from build123d import *

# Parameters (mm, degrees)
F0_R     = 3.675
F0_R_2   = 3.175
F1_DEPTH = 2.38125
F0_R_3   = 6.35
F0_R_4   = 5.85
F3_R     = 5.85
F3_R_2   = 3.675
F4_DEPTH = 0.25


# Not quite as in the source:
# - a length typed as a fraction of an inch, garbled in the dataset ("3 / 203.2 mm" for 3/8 in), is restored


with BuildPart() as f1:
    # F0 (on Top) → F1 (new body, symmetric)
    with BuildSketch(Plane.XY):
        Circle(F0_R)
        Circle(F0_R_2, mode=Mode.SUBTRACT)
    extrude(amount=F1_DEPTH, both=True)



with BuildPart() as f1b:
    # F0 (on Top) → F1, piece 2 (new body, symmetric)
    with BuildSketch(Plane.XY):
        Circle(F0_R_3)
        Circle(F0_R_4, mode=Mode.SUBTRACT)
    extrude(amount=F1_DEPTH, both=True)


with BuildPart() as f1_1:
    add(f1.part)

    add(f1b.part)  # F4 merges F1b
    # F3 (on offset) → F4 (join)
    with BuildSketch(Plane.XY.offset(1.88125)):
        Circle(F3_R)
        Circle(F3_R_2, mode=Mode.SUBTRACT)
    extrude(amount=F4_DEPTH)

    # F5: F1 across plane


with BuildPart() as f1_2:
    add(f1_1.part)
    add(f1_1.part.mirror(Plane.XY))


solid = f1_2.part
Design review of the part built by this model. Coordinates are the model's own, in mm. A direction names the side the tool comes from. Round coordinates to 2 decimals unless told otherwise and drop trailing zeros. Order: outer loops, then holes, each group sorted by start corner. A loop starts at its lowest first (then second) coordinate and runs counter-clockwise, first axis right, second up.
1) Clearance check with a flat-ended pin moving along its axis: pin 1 Ø4 at (x, y) = (0.5, 1) entering from -Z. State where the tip first meets the part, or that it passes through.
The answers:
pin 1: passes through
2) Consider section A-A (y = 0). Count the separate pieces of the cut face and the enclosed holes in it, plus the area to 3 significant figures.
The answers:
separate pieces: 2
enclosed holes: 2
area: 11.7 mm2
3) Consider section C-C (z = -1.7). State the section outline as (x, y) points (3 decimals).
The answers:
outline: circle Ø12.7 at (0, 0); circle Ø7.35 at (0, 0); hole circle Ø11.7 at (0, 0); hole circle Ø6.35 at (0, 0)
4) Draft analysis for pull direction Z (two halves, no side actions). For faces 1 (the cylindrical face through (-1.27, -5.71, -0.03)), 2 (the cylindrical face through (-0.69, -3.1, -0.03)), 3 (the cylindrical face through (-0.797, -3.588, 0.026)), 4 (the flat face through (-3, -3, -2.131)), state which applies: released by +Z, released by -Z, zero draft, split by the parting line, or undercut.
The answers:
face 1: undercut
face 2: zero draft
face 3: undercut
face 4: released by -Z
5) For L1, parallel to Y at x = 0, z = -2.25 (3 decimals); L2, parallel to Z at x = -0.5, y = 3.75; L3, parallel to X at y = 0.25, z = -0.8, list the stretches that pass through material, from the lowest coordinate up.
The answers:
L1: y = -6.35 to -5.85, -3.675 to -3.175, 3.175 to 3.675, 5.85 to 6.35
L2: z = -2.13 to -1.88, 1.88 to 2.13
L3: x = -6.35 to -5.84, -3.67 to -3.17, 3.17 to 3.67, 5.84 to 6.35
6) Consider section D-D (y = -4). State the section outline as (x, z) points, plus the area to 3 significant figures.
The answers:
outline: (-4.93, -2.38) - (-4.27, -2.38) - (-4.27, -2.13) - (4.27, -2.13) - (4.27, -2.38) - (4.93, -2.38) - (4.93, 2.38) - (4.27, 2.38) - (4.27, 2.13) - (-4.27, 2.13) - (-4.27, 2.38) - (-4.93, 2.38) - close; hole (-4.27, -1.88) - (4.27, -1.88) - (4.27, 1.88) - (-4.27, 1.88) - close
area: 10.6 mm2
7) Machinability: for faces 5 (the flat face through (-3, -3, 2.131)), 6 (the flat face through (-3, -3, -1.881)), 7 (the cylindrical face through (-1.38, -6.2, 0.03)), which of the approach directions +Z, -Z, +X, -X, +Y, -Y give a long, thin tool a straight path to every point of the face, cutting with its end or side? Answer none if there is none.
The answers:
face 5: +Z
face 6: none
face 7: +Z, -Z
